```python
from build123d import *

# Parameters (mm, degrees)
EXTRUDE_1_DEPTH     = 20
CHAMFER_1_SIZE      = 2
CHAMFER_3_SIZE      = 0.5
SKETCH_2_R          = 4
EXTRUDE_2_DEPTH     = 3
SKETCH_3_R          = 1.5
CUT_EXTRUDE_1_DEPTH = 10


with BuildPart() as part:
    # 草图1 → 凸台-拉伸1 (new body)
    with BuildSketch(Plane(origin=(0, 0, 0), x_dir=(1, 0, 0), z_dir=(0, 1, 0))):
        Polygon((-7, 12.6), (0, 12.6), (0, -12.6), (-7, -12.6), (-7, -7.6), (-3, -7.6), (-3, 7.6), (-7, 7.6), align=None)
    extrude(amount=EXTRUDE_1_DEPTH)

    # 倒角1
    chamfer_1_edges = [part.edges().sort_by_distance(p)[0] for p in [
        (0, 10, -12.6),
        (0, 10, 12.6),
    ]]
    chamfer(chamfer_1_edges, length=CHAMFER_1_SIZE)

    # 倒角3
    chamfer_3_edges = [part.edges().sort_by_distance(p)[0] for p in [
        (-7, 10, 7.6),
        (-7, 10, -7.6),
    ]]
    chamfer(chamfer_3_edges, length=CHAMFER_3_SIZE)

    # 草图2 → 凸台-拉伸2 (add)
    with BuildSketch(Plane(origin=(0, 0, 0), x_dir=(0, 0, -1), z_dir=(1, 0, 0))):
        with Locations((0, 10)):
            Circle(SKETCH_2_R)
    extrude(amount=EXTRUDE_2_DEPTH)

    # 草图3 → 切除-拉伸1 (cut)
    with BuildSketch(Plane(origin=(3, 0, 0), x_dir=(0, 0, -1), z_dir=(1, 0, 0))):
        with Locations((0, 10)):
            Circle(SKETCH_3_R)
    extrude(amount=-CUT_EXTRUDE_1_DEPTH, mode=Mode.SUBTRACT)


solid = part.part
```
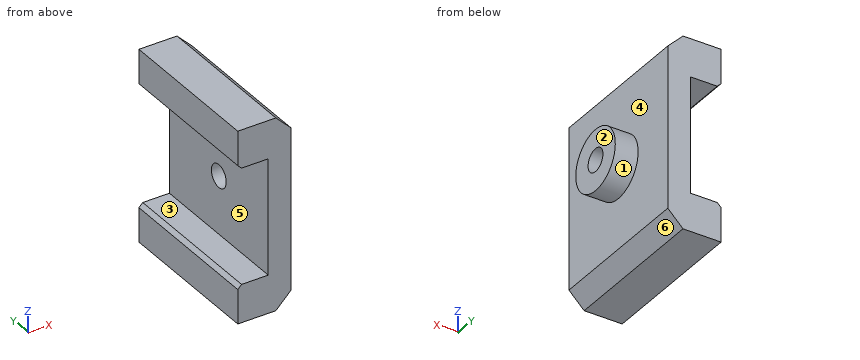
Check sheet for the modelled part. Datum: model origin and axes. Units: mm. Face numbers are marked on the shaded views. A direction names the side the tool comes from. Round coordinates to 2 decimals unless told otherwise and drop trailing zeros. Order: outer loops, then holes, each group sorted by start corner. A loop starts at its lowest first (then second) coordinate and runs counter-clockwise, first axis right, second up. Notation, with made-up numbers: (79.25, 66.5) -> (128.25, 66.5) arc R20 ccw to (128.25, 77.5) -> close; hole circle Ø5 at (5.5, 70). An arc over 180 degrees is marked (long way). One line per item, written item: value. Start each with the question number.
Q1. Set-up check for the marked faces 1, 2 and 3: record each of +Z, -Z, +X, -X, +Y, -Y from which the full face is reachable in a straight line by a thin tool's end or side.
Q2. Mould release check, pull along Z, two halves, no side actions. Record for the marked faces 4, 5 and 6: pulls with the +Z half, pulls with the -Z half, needs draft (parallel to the pull), parting line crosses it, or undercut.
Q3. Cross-section at C-C (y = 10). Record the boundary of the cut face in (x, z), and give its area (3 significant figures).
Q4. Cross-section at D-D (x = 2.25). Record the boundary of the cut face in (y, z), and give its area (3 significant figures).
Q5. Thickness scan on line 1 (Y direction, x = -1.4, z = 0); line 2 (Y direction, x = 1.25, z = 0); line 3 (X direction, y = 11.75, z = -0.25). Record the ranges inside material, lowest first.
Q6. Cross-section at A-A (z = 0). Record the boundary of the cut face in (x, y), and give its area (3 significant figures).
Q7. Cross-section at B-B (x = -4.5). Record the boundary of the cut face in (y, z), and give its area (3 significant figures).
Q8. Gauge pin test, flat ends, axial feed: pin 1 Ø3 at (y, z) = (15.5, -1.5) entering from +X; pin 2 Ø12 at (y, z) = (14.5, 0.5) entering from -X. Record the tip position at first contact, or that the pin passes through.
Completed:
1. face 1: +X
1. face 2: +Z, -Z, +X, +Y, -Y
1. face 3: -X, +Y, -Y
2. face 4: needs draft
2. face 5: undercut
2. face 6: pulls with the -Z half
3. outline: (-7, -12.6) -> (-2, -12.6) -> (0, -10.6) -> (0, -4) -> (3, -4) -> (3, -1.5) -> (-3, -1.5) -> (-3, -7.6) -> (-6.5, -7.6) -> (-7, -8.1) -> close; (-7, 8.1) -> (-6.5, 7.6) -> (-3, 7.6) -> (-3, 1.5) -> (3, 1.5) -> (3, 4) -> (0, 4) -> (0, 10.6) -> (-2, 12.6) -> (-7, 12.6) -> close
3. area: 117 mm²
4. outline: circle Ø8 at (10, 0); hole circle Ø3 at (10, 0)
4. area: 43.2 mm²
5. line 1: y = 0 to 8.5, 11.5 to 20
5. line 2: y = 6 to 8.5, 11.5 to 14
5. line 3: x = -3 to 3
6. outline: (-3, 0) -> (0, 0) -> (0, 6) -> (3, 6) -> (3, 8.5) -> (-3, 8.5) -> close; (-3, 11.5) -> (3, 11.5) -> (3, 14) -> (0, 14) -> (0, 20) -> (-3, 20) -> close
6. area: 66.0 mm²
7. outline: (0, -12.6) -> (20, -12.6) -> (20, -7.6) -> (0, -7.6) -> close; (0, 7.6) -> (20, 7.6) -> (20, 12.6) -> (0, 12.6) -> close
7. area: 200 mm²
8. pin 1: stops at x = 0
8. pin 2: stops at x = -3
